CAD build for the part. Positions are in the model's coordinates, mm. A direction names the side the tool comes from. Give positions to 0.01 mm unless a question says otherwise; leave off trailing zeros. Order: outer loops, then holes, each group sorted by start corner. A loop starts at its lowest first (then second) coordinate and runs counter-clockwise, first axis right, second up.
Item 1: Two-plate mould, pull along X, no slides. Class faces 6 (the flat face through (9, 0, 9)), 7 (the flat face through (2.225, 33, 6)), 8 (the flat face through (0.5, 14, 9)): released by +X, released by -X, zero draft, split by the parting line, or undercut.
Item 2: Band-saw the part on C-C on z = 12.5. Give the cut face in (x, y).
Item 3: Wall check: L1, parallel to X at y = 35.5, z = 4.5 (3 decimals); L2, parallel to X at y = 29.5, z = 6.75; L3, parallel to Y at x = 4.5, z = 13.25. Give the ranges that are in metal, low to high.
Item 4: Flat gauge pins, fed straight in: P1, Ø1.1, axis at x = 17, z = 17, coming from the +Y side; P2, Ø2.5, axis at y = 7.5, z = 8.5, coming from the +X side; P3, Ø3, axis at x = 4, y = 30.5, coming from the +Z side. Where does each tip first touch, or does it go through?
Item 5: Which spindle directions (+Z, -Z, +X, -X, +Y, -Y) get a long thin tool onto all of the face, cutting with end or side? Do faces 1 (the flat face through (16.96, 12.81, 16.83)), 2 (the flat face through (4.225, 33, 6)), 3 (the flat face through (6, 33, 14)), 4 (the flat face through (14, 27.75, 14)), 5 (the flat face through (0.3, 8, 17.1)). Say none if no direction does.
Item 6: Band-saw the part on B-B on y = 16. Give the cut face in (x, z).
Item 7: Band-saw the part on A-A on z = 4.25. Give the cut face in (x, y) (3 decimals).
Item 8: Band-saw the part on D-D on x = 3.5. Give the cut face in (y, z).
```python
from build123d import *

# Parameters (mm, degrees)
SKETCH1_W                      = 17.45
SKETCH1_H                      = 37.75
PROFILEBOSS_EXTRUDE1_DEPTH     = 17.34
TOPINDENTSSKETCH2_W            = 6
TOPINDENTSSKETCH2_H            = 10
TOPINDENTCUT_EXTRUDE1_DEPTH    = 6
MOUNTSLOTCUTCUT_EXTRUDE2_DEPTH = 44.106386998
FRONTEDGECHAMFER1_START        = 8
FRONTEDGECHAMFER1_DEPTH        = 9.75
RIGHTSLOTSKETCH4_W             = 5.34
RIGHTSLOTSKETCH4_H             = 27.610084113
RIGHTSLOTCUT_EXTRUDE5_DEPTH    = 0.5
LEFTSLOTSKETCH5_W              = 5.34
LEFTSLOTSKETCH5_H              = 27.50506845
CUT_EXTRUDE8_DEPTH             = 0.5


with BuildPart() as part:
    # Sketch1 → ProfileBoss-Extrude1 (new body)
    with BuildSketch(Plane.XY):
        with Locations((8.725, 18.875)):
            Rectangle(SKETCH1_W, SKETCH1_H)
    extrude(amount=PROFILEBOSS_EXTRUDE1_DEPTH)

    # TopIndentsSketch2 → TopIndentCut-Extrude1 (cut)
    with BuildSketch(Plane.XY.offset(17.34)):
        with Locations((14.45, 32.75)):
            Rectangle(TOPINDENTSSKETCH2_W, TOPINDENTSSKETCH2_H)
        with Locations((3, 32.75)):
            Rectangle(TOPINDENTSSKETCH2_W, TOPINDENTSSKETCH2_H)
    extrude(amount=-TOPINDENTCUT_EXTRUDE1_DEPTH, mode=Mode.SUBTRACT)

    # Sketch3 → MountSlotCutCut-Extrude2 (cut, through all)
    with BuildSketch(Plane.XY.offset(11.34)):
        with BuildLine():
            Line((13.225, 29.75), (13.225, 35.75))
            ThreePointArc((13.225, 35.75), (14.225, 36.75), (15.225, 35.75))
            Line((15.225, 35.75), (15.225, 29.75))
            ThreePointArc((15.225, 29.75), (14.225, 28.75), (13.225, 29.75))
        make_face()
        with BuildLine():
            Line((2.225, 29.75), (2.225, 35.75))
            ThreePointArc((2.225, 35.75), (3.225, 36.75), (4.225, 35.75))
            Line((4.225, 35.75), (4.225, 29.75))
            ThreePointArc((4.225, 29.75), (3.225, 28.75), (2.225, 29.75))
        make_face()
    extrude(amount=-MOUNTSLOTCUTCUT_EXTRUDE2_DEPTH, mode=Mode.SUBTRACT)

    # FrontEdgeChamfer1: read off the stored shape, not the designer's step
    # FrontEdgeChamfer1 outline → FrontEdgeChamfer1 (cut)
    with BuildSketch(Plane(origin=(0, 0, 0), x_dir=(1, 0, 0), z_dir=(0, 1, 0)).offset(FRONTEDGECHAMFER1_START)):
        Polygon((17.45, -17.34), (17.45, -16.34), (16.45, -17.34), align=None)
        Polygon((0, -17.34), (1, -17.34), (0, -16.34), align=None)
    extrude(amount=FRONTEDGECHAMFER1_DEPTH, mode=Mode.SUBTRACT)

    # RightSlotSketch4 → RightSlotCut-Extrude5 (cut)
    with BuildSketch(Plane(origin=(17.45, 0, 0), x_dir=(0, 0, -1), z_dir=(1, 0, 0))):
        with Locations((-8.67, 13.805042057)):
            Rectangle(RIGHTSLOTSKETCH4_W, RIGHTSLOTSKETCH4_H)
    extrude(amount=-RIGHTSLOTCUT_EXTRUDE5_DEPTH, mode=Mode.SUBTRACT)

    # LeftSlotSketch5 → Cut-Extrude8 (cut)
    with BuildSketch(Plane.ZY):
        with Locations((8.67, 13.752534225)):
            Rectangle(LEFTSLOTSKETCH5_W, LEFTSLOTSKETCH5_H)
    extrude(amount=-CUT_EXTRUDE8_DEPTH, mode=Mode.SUBTRACT)


solid = part.part
```
The answers:
1. face 6: zero draft
1. face 7: undercut
1. face 8: released by -X
2. outline: (0, 0) - (17.45, 0) - (17.45, 27.75) - (11.45, 27.75) - (11.45, 37.75) - (6, 37.75) - (6, 27.75) - (0, 27.75) - close
3. L1: x = 0 to 2.225, 4.225 to 13.225, 15.225 to 17.45
3. L2: x = 0 to 2.26, 4.19 to 13.26, 15.19 to 17.45
3. L3: y = 0 to 27.75
4. P1: stops at y = 27.75
4. P2: stops at x = 16.95
4. P3: stops at z = 11.34
5. face 1: +Z, +X
5. face 2: +Z, -Z
5. face 3: +Z, -X, +Y
5. face 4: +Z, +X, +Y
5. face 5: +Z, -X
6. outline: (0, 0) - (17.45, 0) - (17.45, 6) - (16.95, 6) - (16.95, 11.34) - (17.45, 11.34) - (17.45, 16.34) - (16.45, 17.34) - (1, 17.34) - (0, 16.34) - (0, 11.34) - (0.5, 11.34) - (0.5, 6) - (0, 6) - close
7. outline: (0, 0) - (17.45, 0) - (17.45, 37.75) - (0, 37.75) - close; hole (2.225, 29.75) arc R1 ccw to (4.225, 29.75) - (4.225, 35.75) arc R1 ccw to (2.225, 35.75) - close; hole (13.225, 29.75) arc R1 ccw to (15.225, 29.75) - (15.225, 35.75) arc R1 ccw to (13.225, 35.75) - close
8. outline: (0, 0) - (28.79, 0) - (28.79, 11.34) - (27.75, 11.34) - (27.75, 17.34) - (0, 17.34) - close; (36.71, 0) - (37.75, 0) - (37.75, 11.34) - (36.71, 11.34) - close
